```python
from build123d import *

# Parameters (mm, degrees)
F1_DEPTH  = 25
F2_R      = 1.1
F3_DEPTH  = 32.301
F4_R      = 1.1
F4_R_2    = 4
F5_DEPTH  = 1.5
F6_R      = 1
F7_W      = 29.3
F7_H      = 1.5
F8_DEPTH  = 4
F9_W      = 29.3
F9_H      = 1.5
F10_DEPTH = 30.8
F11_W     = 29.3
F11_H     = 1.5
F12_DEPTH = 20
F13_R     = 1.1
F14_DEPTH = 1.5
F16_DEPTH = 30.8


with BuildPart() as f1:
    # F0 (on Front) → F1 (new body)
    with BuildSketch(Plane.XZ):
        Polygon((0, 19.5), (0, 0), (1.5, 0), (1.5, 18), (30.8, 18), (30.8, 0), (32.3, 0), (32.3, 19.5), align=None)
    extrude(amount=F1_DEPTH)

    # F2 (on face) → F3 (cut, through all)
    with BuildSketch(Plane(origin=(0, 0, 0), x_dir=(0, -1, 0), z_dir=(-1, 0, 0))):
        with BuildLine():
            Line((16.5, 0), (16.5, 2))
            ThreePointArc((16.5, 2), (12.5, 6), (8.5, 2))
            Line((8.5, 2), (8.5, 0))
            Line((8.5, 0), (16.5, 0))
        make_face()
        with Locations((18.7225396744, 2)):
            Circle(F2_R)
        with Locations((16.9, 6.4)):
            Circle(F2_R)
        with Locations((12.5, 8.2225396744)):
            Circle(F2_R)
        with Locations((8.1, 6.4)):
            Circle(F2_R)
        with Locations((6.2774603256, 2)):
            Circle(F2_R)
        Polygon((0, 0), (3.2774603256, 0), (0.4682086179, 18), (0, 18), align=None)
        Polygon((21.7225396744, 0), (25, 0), (25, 18), (24.5317913821, 18), align=None)
    extrude(amount=-F3_DEPTH, mode=Mode.SUBTRACT)

    # F4 (on face) → F5 (cut, through all)
    with BuildSketch(Plane.XY.offset(19.5)):
        with Locations((6.15, -2.5)):
            Circle(F4_R)
        with Locations((26.15, -2.5)):
            Circle(F4_R)
        with Locations((6.15, -22.5)):
            Circle(F4_R)
        with Locations((26.15, -22.5)):
            Circle(F4_R)
        with Locations((16.15, -12.5)):
            Circle(F4_R_2)
        with Locations((11.75, -8.1)):
            Circle(F4_R)
        with Locations((9.9274603256, -12.5)):
            Circle(F4_R)
        with Locations((11.75, -16.9)):
            Circle(F4_R)
        with Locations((16.15, -18.7225396744)):
            Circle(F4_R)
        with Locations((20.55, -16.9)):
            Circle(F4_R)
        with Locations((22.3725396744, -12.5)):
            Circle(F4_R)
        with Locations((20.55, -8.1)):
            Circle(F4_R)
        with Locations((16.15, -6.2774603256)):
            Circle(F4_R)
    extrude(amount=-F5_DEPTH, mode=Mode.SUBTRACT)

    # F6
    f6_edges = [f1.edges().sort_by_distance(p)[0] for p in [
        (31.55, -3.27746, 0),
        (0.75, -3.27746, 0),
        (31.55, -8.5, 0),
        (0.75, -8.5, 0),
        (31.55, -16.5, 0),
        (0.75, -16.5, 0),
        (31.55, -21.72254, 0),
        (0.75, -21.72254, 0),
    ]]
    fillet(f6_edges, radius=F6_R)

    # F7 (on face) → F8 (join)
    with BuildSketch(Plane(origin=(0, 0, 0), x_dir=(-1, 0, 0), z_dir=(0, 1, 0))):
        with Locations((-16.15, 18.75)):
            Rectangle(F7_W, F7_H)
    extrude(amount=F8_DEPTH)

    # F9 (on face) → F10 (join)
    with BuildSketch(Plane.XY.offset(19.5)):
        with Locations((16.15, 3.25)):
            Rectangle(F9_W, F9_H)
    extrude(amount=F10_DEPTH)

    # F11 (on face) → F12 (join)
    with BuildSketch(Plane.XZ.offset(-2.5)):
        with Locations((16.15, 49.55)):
            Rectangle(F11_W, F11_H)
    extrude(amount=F12_DEPTH)

    # F13 (on face) → F14 (cut, through all)
    with BuildSketch(Plane(origin=(0, 0, 48.8), x_dir=(1, 0, 0), z_dir=(0, 0, -1))):
        with Locations((9.9274603256, 12.5)):
            Circle(F13_R)
        with Locations((11.75, 8.1)):
            Circle(F13_R)
        with Locations((16.15, 6.2774603256)):
            Circle(F13_R)
        with Locations((20.55, 8.1)):
            Circle(F13_R)
        with Locations((22.3725396744, 12.5)):
            Circle(F13_R)
        with BuildLine():
            Line((12.15, 15), (12.15, 12.5))
            ThreePointArc((12.15, 12.5), (16.15, 8.5), (20.15, 12.5))
            Line((20.15, 12.5), (20.15, 15))
            Line((20.15, 15), (25.8, 15))
            Line((25.8, 15), (30.8, -2.5))
            Line((30.8, -2.5), (30.8, 17.5))
            Line((30.8, 17.5), (1.5, 17.5))
            Line((1.5, 17.5), (1.5, -2.5))
            Line((1.5, -2.5), (6.5, 15))
            Line((6.5, 15), (12.15, 15))
        make_face()
    extrude(amount=-F14_DEPTH, mode=Mode.SUBTRACT)

    # F15 (on face) → F16 (cut)
    with BuildSketch(Plane.XY.offset(50.3)):
        Polygon((1.5, 2.5), (4.5285714286, -8.1), (4.5285714286, 4), (1.5, 4), align=None)
        Polygon((30.8, 4), (27.7714285714, 4), (27.7714285714, -8.1), (30.8, 2.5), align=None)
    extrude(amount=-F16_DEPTH, mode=Mode.SUBTRACT)


solid = f1.part
```
Model file for the job. Use its own axes, mm. A direction names the side the tool comes from. Give positions to 0.01 mm unless a question says otherwise; leave off trailing zeros. Order: outer loops, then holes, each group sorted by start corner. A loop starts at its lowest first (then second) coordinate and runs counter-clockwise, first axis right, second up.
1) Saw through at A-A, the plane x = 22.5. Write the cut outline in (y, z).
2) Saw through at B-B, the plane y = -22.5. Write the cut outline in (x, z), then the cut area to 3 significant figures.
3) Saw through at D-D, the plane z = 29. Write the cut outline in (x, y), then the cut area to 3 significant figures.
4) Saw through at C-C, the plane z = 16. Write the cut outline in (x, y).
5) Mould opens along Z. For faces 4 (the cylindrical face through (31.56, -16.801, 0.285)), 5 (the cylindrical face through (31.54, -17.916, 5.979)), 6 (the cylindrical face through (0.74, -7.294, 1.579)), 7 (the flat face through (16, -3, 50.3)) say: +Z half, -Z half, draft (parallel to the pull), parting line (faces both ways), or undercut.
6) Pin check, flat tips, straight feed: pin 1 (2 mm diameter, centred on x = 3.5, y = -1, fed in from -Z); pin 2 (1.8 mm diameter, centred on y = -18.72, z = 2, fed in from +X); pin 3 (6 mm diameter, centred on y = -11.5, z = 19, fed in from -X); pin 4 (6 mm diameter, centred on x = 25, z = 34.5, fed in from -Y). Stop position of each tip, or through.
7) Wall check: probe 1 along X at (y, z) = (-2, 13); probe 2 along Z at (x, y) = (20.5, 1); probe 3 along Z at (x, y) = (7.5, -20). Give the ranges that are in metal, low to high.
8) 3-axis set-ups, long thin cutter, end or side, ignore diameter. For faces 1 (the flat face through (30.8, -12, 11)), 2 (the flat face through (12.15, -14, 50)), 3 (the flat face through (5.5, -11.5, 49.5)): which of +Z, -Z, +X, -X, +Y, -Y reach the whole face in a straight line?
Computed:
1. outline: (-25, 18) - (-13.59, 18) - (-13.59, 19.5) - (-25, 19.5) - close; (-15, 48.8) - (-13.59, 48.8) - (-13.59, 50.3) - (-15, 50.3) - close; (-11.41, 18) - (4, 18) - (4, 50.3) - (-11.41, 50.3) - (-11.41, 48.8) - (2.5, 48.8) - (2.5, 19.5) - (-11.41, 19.5) - close
2. outline: (0, 4.98) - (1.5, 4.98) - (1.5, 18) - (5.05, 18) - (5.05, 19.5) - (0, 19.5) - close; (7.25, 18) - (25.05, 18) - (25.05, 19.5) - (7.25, 19.5) - close; (27.25, 18) - (30.8, 18) - (30.8, 4.98) - (32.3, 4.98) - (32.3, 19.5) - (27.25, 19.5) - close
2. area: 80.9 mm2
3. outline: (4.53, 2.5) - (27.77, 2.5) - (27.77, 4) - (4.53, 4) - close
3. area: 34.9 mm2
4. outline: (0, -24.22) - (1.5, -24.22) - (1.5, -0.78) - (0, -0.78) - close; (30.8, -24.22) - (32.3, -24.22) - (32.3, -0.78) - (30.8, -0.78) - close
5. face 4: -Z half
5. face 5: undercut
5. face 6: undercut
5. face 7: +Z half
6. pin 1: stops at z = 18
6. pin 2: passes through
6. pin 3: stops at x = 0
6. pin 4: stops at y = 2.5
7. probe 1: x = 0 to 1.5, 30.8 to 32.3
7. probe 2: z = 18 to 19.5, 48.8 to 50.3
7. probe 3: z = 18 to 19.5
8. face 1: -Z, +Y, -Y
8. face 2: +Z, -Y
8. face 3: +Z, -X, -Y
